Here's how the part is built. I have some questions about the finished solid (model axes, mm). A direction names the side the tool comes from. Give positions to 0.01 mm unless a question says otherwise; leave off trailing zeros. Loops run counter-clockwise (first coordinate to the right, second up) from the corner with the lowest first, then second, coordinate; pieces in that order, holes last. Notation, with made-up numbers: M 24,20 L 55,20 A19 cw 55,55 Z; hole C 75.25,83.5 d10. An arc over 180 degrees is marked long. Write item = value, one per line. Start each with the question number.
```python
from build123d import *
from build123d.topology import SkipClean

# Parameters (mm, degrees)
SKETCH_1_R           = 25
EXTRUDE_1_DEPTH      = 22
SKETCH_2_W           = 140
SKETCH_2_H           = 100
EXTRUDE_2_DEPTH      = 10
SKETCH_4_W           = 140
SKETCH_4_H           = 20
EXTRUDE_3_DEPTH      = 150
CUT_EXTRUDE_1_DEPTH  = 150
CUT_EXTRUDE_3_REACH  = 221.144
SKETCH_8_R           = 50
CUT_EXTRUDE_4_REACH  = 221.144
SKETCH_9_R           = 45
SKETCH_7_R           = 4.5
EXTRUDE_4_DEPTH      = 50
CUT_EXTRUDE_5_REACH  = 221.144
SKETCH_10_R          = 2.5
CUT_EXTRUDE_START    = -5
SKETCH_11_R          = 4
SKETCH_11_R_2        = 2.5
CUT_EXTRUDE_7_DEPTH  = 5
CUT_EXTRUDE_9_REACH  = 221.144
SKETCH_13_R          = 2.5
SKETCH_14_R          = 4
CUT_EXTRUDE_11_DEPTH = 5
SKETCH_16_W          = 6
SKETCH_16_H          = 3
EXTRUDE_5_DEPTH      = 50
CUT_EXTRUDE_12_DEPTH = 30


with BuildPart() as part:
    # 草图1 → 凸台-拉伸1 (new body)
    with BuildSketch(Plane.XY):
        with Locations((0, -0.593277016)):
            Circle(SKETCH_1_R)
    extrude(amount=EXTRUDE_1_DEPTH)

    # 草图2 → 凸台-拉伸2 (add)
    with BuildSketch(Plane.XY.offset(22)):
        Rectangle(SKETCH_2_W, SKETCH_2_H)
    extrude(amount=EXTRUDE_2_DEPTH)

    # 草图4 → 凸台-拉伸3 (add)
    with BuildSketch(Plane.XY.offset(32)):
        with Locations((0, 40)):
            Rectangle(SKETCH_4_W, SKETCH_4_H)
        with Locations((0, -40)):
            Rectangle(SKETCH_4_W, SKETCH_4_H)
    extrude(amount=EXTRUDE_3_DEPTH)

    # 草图6 → 切除-拉伸1 (cut)
    with BuildSketch(Plane(origin=(0, 50, 0), x_dir=(1, 0, 0), z_dir=(0, 1, 0))):
        with BuildLine():
            ThreePointArc((0, -182), (-49.497474683, -161.497474683), (-70, -112))
            Line((-70, -112), (-70, -182))
            Line((-70, -182), (0, -182))
        make_face()
        with BuildLine():
            Line((70, -182), (70, -112))
            ThreePointArc((70, -112), (49.497474683, -161.497474683), (0, -182))
            Line((0, -182), (70, -182))
        make_face()
    extrude(amount=-CUT_EXTRUDE_1_DEPTH, mode=Mode.SUBTRACT)

    # 草图8 → 切除-拉伸3 (cut, up to next)
    with BuildSketch(Plane(origin=(0, 50, 0), x_dir=(1, 0, 0), z_dir=(0, 1, 0)), mode=Mode.PRIVATE) as cut_extrude_3_sk1:
        with Locations(Location((0, -112, 0), (0, 0, 270))):
            Circle(SKETCH_8_R)
    cut_extrude_3_tool1 = extrude(cut_extrude_3_sk1.sketch, amount=-CUT_EXTRUDE_3_REACH, mode=Mode.PRIVATE) & part.part
    add(cut_extrude_3_tool1.solids().sort_by_distance((0, 50, 112))[0], mode=Mode.SUBTRACT)

    # 草图9 → 切除-拉伸4 (cut, up to next)
    with BuildSketch(Plane.XZ.offset(50), mode=Mode.PRIVATE) as cut_extrude_4_sk1:
        with Locations(Location((0, 112, 0), (0, 0, 270))):
            Circle(SKETCH_9_R)
    cut_extrude_4_tool1 = extrude(cut_extrude_4_sk1.sketch, amount=-CUT_EXTRUDE_4_REACH, mode=Mode.PRIVATE) & part.part
    add(cut_extrude_4_tool1.solids().sort_by_distance((0, -50, 112))[0], mode=Mode.SUBTRACT)

    # 草图7 → 凸台-拉伸4 (add)
    with BuildSketch(Plane(origin=(0, 0, 0), x_dir=(-1, 0, 0), z_dir=(0, 0, -1))):
        Circle(SKETCH_7_R)
    extrude(amount=EXTRUDE_4_DEPTH)

    # 草图10 → 切除-拉伸5 (cut, up to next)
    with BuildSketch(Plane.XZ.offset(50), mode=Mode.PRIVATE) as cut_extrude_5_sk1:
        with Locations(Location((0, 172, 0), (0, 0, 270))):
            Circle(SKETCH_10_R)
    cut_extrude_5_tool1 = extrude(cut_extrude_5_sk1.sketch, amount=-CUT_EXTRUDE_5_REACH, mode=Mode.PRIVATE) & part.part
    # 草图10 → 切除-拉伸5 (cut, up to next)
    with BuildSketch(Plane.XZ.offset(50), mode=Mode.PRIVATE) as cut_extrude_5_sk2:
        with Locations(Location((51.961524227, 142, 0), (0, 0, 270))):
            Circle(SKETCH_10_R)
    cut_extrude_5_tool2 = extrude(cut_extrude_5_sk2.sketch, amount=-CUT_EXTRUDE_5_REACH, mode=Mode.PRIVATE) & part.part
    # 草图10 → 切除-拉伸5 (cut, up to next)
    with BuildSketch(Plane.XZ.offset(50), mode=Mode.PRIVATE) as cut_extrude_5_sk3:
        with Locations(Location((51.961524227, 82, 0), (0, 0, 270))):
            Circle(SKETCH_10_R)
    cut_extrude_5_tool3 = extrude(cut_extrude_5_sk3.sketch, amount=-CUT_EXTRUDE_5_REACH, mode=Mode.PRIVATE) & part.part
    # 草图10 → 切除-拉伸5 (cut, up to next)
    with BuildSketch(Plane.XZ.offset(50), mode=Mode.PRIVATE) as cut_extrude_5_sk4:
        with Locations(Location((0, 52, 0), (0, 0, 270))):
            Circle(SKETCH_10_R)
    cut_extrude_5_tool4 = extrude(cut_extrude_5_sk4.sketch, amount=-CUT_EXTRUDE_5_REACH, mode=Mode.PRIVATE) & part.part
    # 草图10 → 切除-拉伸5 (cut, up to next)
    with BuildSketch(Plane.XZ.offset(50), mode=Mode.PRIVATE) as cut_extrude_5_sk5:
        with Locations(Location((-51.961524227, 82, 0), (0, 0, 270))):
            Circle(SKETCH_10_R)
    cut_extrude_5_tool5 = extrude(cut_extrude_5_sk5.sketch, amount=-CUT_EXTRUDE_5_REACH, mode=Mode.PRIVATE) & part.part
    # 草图10 → 切除-拉伸5 (cut, up to next)
    with BuildSketch(Plane.XZ.offset(50), mode=Mode.PRIVATE) as cut_extrude_5_sk6:
        with Locations(Location((-51.961524227, 142, 0), (0, 0, 270))):
            Circle(SKETCH_10_R)
    cut_extrude_5_tool6 = extrude(cut_extrude_5_sk6.sketch, amount=-CUT_EXTRUDE_5_REACH, mode=Mode.PRIVATE) & part.part
    add(cut_extrude_5_tool1.solids().sort_by_distance((0, -50, 172))[0], mode=Mode.SUBTRACT)
    add(cut_extrude_5_tool2.solids().sort_by_distance((51.961524, -50, 142))[0], mode=Mode.SUBTRACT)
    add(cut_extrude_5_tool3.solids().sort_by_distance((51.961524, -50, 82))[0], mode=Mode.SUBTRACT)
    add(cut_extrude_5_tool4.solids().sort_by_distance((0, -50, 52))[0], mode=Mode.SUBTRACT)
    add(cut_extrude_5_tool5.solids().sort_by_distance((-51.961524, -50, 82))[0], mode=Mode.SUBTRACT)
    add(cut_extrude_5_tool6.solids().sort_by_distance((-51.961524, -50, 142))[0], mode=Mode.SUBTRACT)

    # 草图11 → 切除-拉伸7 (cut)
    # profile 1 of 6: a face of its own
    with BuildSketch(Plane(origin=(0, -30, 0), x_dir=(1, 0, 0), z_dir=(0, 1, 0)).offset(CUT_EXTRUDE_START)):
        with Locations(Location((0, -52, 0), (0, 0, 270))):
            Circle(SKETCH_11_R)
        with Locations(Location((0, -52, 0), (0, 0, 90))):
            Circle(SKETCH_11_R_2, mode=Mode.SUBTRACT)
    # profile 2 of 6: a face of its own
    with BuildSketch(Plane(origin=(0, -30, 0), x_dir=(1, 0, 0), z_dir=(0, 1, 0)).offset(CUT_EXTRUDE_START)):
        with Locations(Location((51.961524227, -82, 0), (0, 0, 270))):
            Circle(SKETCH_11_R)
    # profile 3 of 6: a face of its own
    with BuildSketch(Plane(origin=(0, -30, 0), x_dir=(1, 0, 0), z_dir=(0, 1, 0)).offset(CUT_EXTRUDE_START)):
        with Locations(Location((-51.961524227, -82, 0), (0, 0, 270))):
            Circle(SKETCH_11_R)
    # profile 4 of 6: a face of its own
    with BuildSketch(Plane(origin=(0, -30, 0), x_dir=(1, 0, 0), z_dir=(0, 1, 0)).offset(CUT_EXTRUDE_START)):
        with Locations(Location((-51.961524227, -142, 0), (0, 0, 270))):
            Circle(SKETCH_11_R)
    # profile 5 of 6: a face of its own
    with BuildSketch(Plane(origin=(0, -30, 0), x_dir=(1, 0, 0), z_dir=(0, 1, 0)).offset(CUT_EXTRUDE_START)):
        with Locations(Location((0, -172, 0), (0, 0, 270))):
            Circle(SKETCH_11_R)
    # profile 6 of 6: a face of its own
    with BuildSketch(Plane(origin=(0, -30, 0), x_dir=(1, 0, 0), z_dir=(0, 1, 0)).offset(CUT_EXTRUDE_START)):
        with Locations(Location((51.961524227, -142, 0), (0, 0, 270))):
            Circle(SKETCH_11_R)
    extrude(amount=CUT_EXTRUDE_7_DEPTH, mode=Mode.SUBTRACT)

    # 草图13 → 切除-拉伸9 (cut, up to next)
    with BuildSketch(Plane(origin=(0, 50, 0), x_dir=(1, 0, 0), z_dir=(0, 1, 0)), mode=Mode.PRIVATE) as cut_extrude_9_sk1:
        with Locations(Location((51.961524227, -82, 0), (0, 0, 90))):
            Circle(SKETCH_13_R)
    cut_extrude_9_tool1 = extrude(cut_extrude_9_sk1.sketch, amount=-CUT_EXTRUDE_9_REACH, mode=Mode.PRIVATE) & part.part
    # 草图13 → 切除-拉伸9 (cut, up to next)
    with BuildSketch(Plane(origin=(0, 50, 0), x_dir=(1, 0, 0), z_dir=(0, 1, 0)), mode=Mode.PRIVATE) as cut_extrude_9_sk2:
        with Locations(Location((51.961524227, -142, 0), (0, 0, 90))):
            Circle(SKETCH_13_R)
    cut_extrude_9_tool2 = extrude(cut_extrude_9_sk2.sketch, amount=-CUT_EXTRUDE_9_REACH, mode=Mode.PRIVATE) & part.part
    # 草图13 → 切除-拉伸9 (cut, up to next)
    with BuildSketch(Plane(origin=(0, 50, 0), x_dir=(1, 0, 0), z_dir=(0, 1, 0)), mode=Mode.PRIVATE) as cut_extrude_9_sk3:
        with Locations(Location((0, -172, 0), (0, 0, 90))):
            Circle(SKETCH_13_R)
    cut_extrude_9_tool3 = extrude(cut_extrude_9_sk3.sketch, amount=-CUT_EXTRUDE_9_REACH, mode=Mode.PRIVATE) & part.part
    # 草图13 → 切除-拉伸9 (cut, up to next)
    with BuildSketch(Plane(origin=(0, 50, 0), x_dir=(1, 0, 0), z_dir=(0, 1, 0)), mode=Mode.PRIVATE) as cut_extrude_9_sk4:
        with Locations(Location((-51.961524227, -142, 0), (0, 0, 90))):
            Circle(SKETCH_13_R)
    cut_extrude_9_tool4 = extrude(cut_extrude_9_sk4.sketch, amount=-CUT_EXTRUDE_9_REACH, mode=Mode.PRIVATE) & part.part
    # 草图13 → 切除-拉伸9 (cut, up to next)
    with BuildSketch(Plane(origin=(0, 50, 0), x_dir=(1, 0, 0), z_dir=(0, 1, 0)), mode=Mode.PRIVATE) as cut_extrude_9_sk5:
        with Locations(Location((-51.961524227, -82, 0), (0, 0, 90))):
            Circle(SKETCH_13_R)
    cut_extrude_9_tool5 = extrude(cut_extrude_9_sk5.sketch, amount=-CUT_EXTRUDE_9_REACH, mode=Mode.PRIVATE) & part.part
    add(cut_extrude_9_tool1.solids().sort_by_distance((51.961524, 50, 82))[0], mode=Mode.SUBTRACT)
    add(cut_extrude_9_tool2.solids().sort_by_distance((51.961524, 50, 142))[0], mode=Mode.SUBTRACT)
    add(cut_extrude_9_tool3.solids().sort_by_distance((0, 50, 172))[0], mode=Mode.SUBTRACT)
    add(cut_extrude_9_tool4.solids().sort_by_distance((-51.961524, 50, 142))[0], mode=Mode.SUBTRACT)
    add(cut_extrude_9_tool5.solids().sort_by_distance((-51.961524, 50, 82))[0], mode=Mode.SUBTRACT)

    # 草图14 → 切除-拉伸11 (cut)
    with BuildSketch(Plane.XZ.offset(-30)):
        with Locations(Location((0, 172, 0), (0, 0, 90))):
            Circle(SKETCH_14_R)
        with Locations(Location((-51.961524227, 142, 0), (0, 0, 90))):
            Circle(SKETCH_14_R)
        with Locations(Location((-51.961524227, 82, 0), (0, 0, 90))):
            Circle(SKETCH_14_R)
        with Locations(Location((0, 52, 0), (0, 0, 90))):
            Circle(SKETCH_14_R)
        with Locations(Location((51.961524227, 82, 0), (0, 0, 90))):
            Circle(SKETCH_14_R)
        with Locations(Location((51.961524227, 142, 0), (0, 0, 90))):
            Circle(SKETCH_14_R)
    extrude(amount=-CUT_EXTRUDE_11_DEPTH, mode=Mode.SUBTRACT)

    # 草图16 → 凸台-拉伸5 (add)
    with BuildSketch(Plane(origin=(0, 0, 0), x_dir=(-1, 0, 0), z_dir=(0, 0, -1))):
        with Locations((3, 0)):
            Rectangle(SKETCH_16_W, SKETCH_16_H)
    extrude(amount=EXTRUDE_5_DEPTH)

    # 草图17 → 切除-拉伸12 (cut)
    with SkipClean():  # the faces are left unmerged after this step: merging them gives an invalid solid
        with BuildSketch(Plane(origin=(0, 0, 0), x_dir=(-1, 0, 0), z_dir=(0, 0, -1))):
            with BuildLine():
                Line((6, -1.5), (6, 1.5))
                Line((6, 1.5), (4.242640687, 1.5))
                ThreePointArc((4.242640687, 1.5), (4.435193518, 0.760958904), (4.5, 0))
                ThreePointArc((4.5, 0), (4.435193518, -0.760958904), (4.242640687, -1.5))
                Line((4.242640687, -1.5), (6, -1.5))
            make_face()
        extrude(amount=CUT_EXTRUDE_12_DEPTH, mode=Mode.SUBTRACT)


solid = part.part
```
Q1. If we section it at B-B, the plane z = 172: List the corners of the cut face in (x, y) for me.
Q2. We'd pull the mould along X, two halves only. Please class faces 6 (the flat face through (0, -6, 0)), 7 (the cylindrical face through (50.76, 32.465, 145.815)), 8 (the cylindrical face through (23.846, 6.916, 10.846)): pulls with the +X half, pulls with the -X half, needs draft (parallel to the pull), parting line crosses it, or undercut.
Q3. Will these pins go through, and if not, where does the flat tip stop? pin 1 (12 mm diameter, centred on x = -43, z = 13.5, fed in from +Y); pin 2 (12 mm diameter, centred on x = -51, y = -12.5, fed in from +Z); pin 3 (4 mm diameter, centred on x = -31, y = 22, fed in from -Z); pin 4 (5 mm diameter, centred on y = -37, z = 152.5, fed in from +X).
Q4. If we section it at A-A, the plane x = 36.5: List the corners of the cut face in (y, z) for me.
Q5. If I drill on line 1 along X through (y, z) = (-33.5, 114); line 2 along Y through (x, z) = (-44, 72); line 3 along X through (y, z) = (34.5, 112), over which ranges is the centre line in solid material (lowest first)?
Q6. On a 3-axis mill with a long thin cutter (end or side, diameter ignored), from which of +Z, -Z, +X, -X, +Y, -Y can I reach the whole of each face in a straight line? I mean faces 1 (the cylindrical face through (-0.96, -42.6, 49.69)), 2 (the flat face through (-32, -30, 73)), 3 (the flat face through (-54, -35, 140)), 4 (the cylindrical face through (-54.402, -42.605, 82.542)), 5 (the cylindrical face through (2.2, 40.14, 62.05)). Say none if no direction works.
Q7. If we section it at D-D, the plane y = 22: List the corners of the cut face in (x, z) for me.
Q8. If we section it at C-C, the plane y = 39.5: List the corners of the cut face in (x, z) for me.
Resolved:
q1.outline = M -36.06,-50 L -2.5,-50 L -2.5,-35 L -4,-35 L -4,-30 L -36.06,-30 Z; M -36.06,30 L -4,30 L -4,35 L -2.5,35 L -2.5,50 L -36.06,50 Z; M 2.5,-50 L 36.06,-50 L 36.06,-30 L 4,-30 L 4,-35 L 2.5,-35 Z; M 2.5,35 L 4,35 L 4,30 L 36.06,30 L 36.06,50 L 2.5,50 Z
q2.face_6 = needs draft
q2.face_7 = undercut
q2.face_8 = parting line crosses it
q3.pin_1 = through
q3.pin_2 = 32
q3.pin_3 = 22
q3.pin_4 = 58.79
q4.outline = M -50,22 L 50,22 L 50,77.83 L 30,77.83 L 30,32 L -30,32 L -30,85.68 L -50,85.68 Z; M -50,138.32 L -30,138.32 L -30,171.73 L -50,171.73 Z; M 30,146.17 L 50,146.17 L 50,171.73 L 30,171.73 Z
q5.line_1 = -69.97 to -44.96, 44.96 to 69.97
q5.line_2 = -50 to -30, 30 to 50
q5.line_3 = -70 to -50, 50 to 70
q6.face_1 = -Y
q6.face_2 = +Z, +X, -X
q6.face_3 = none
q6.face_4 = +Y, -Y
q6.face_5 = +Y
q7.outline = M -70,22 L -10.7,22 L -10.7,0 L 10.7,0 L 10.7,22 L 70,22 L 70,32 L -70,32 Z
q8.outline = M -70,22 L 70,22 L 70,112 A70 ccw -70,112 Z; hole C -51.96,82 d5; hole C -51.96,142 d5; hole C 0,112 d100; hole C 0,172 d5; hole C 51.96,82 d5; hole C 51.96,142 d5
